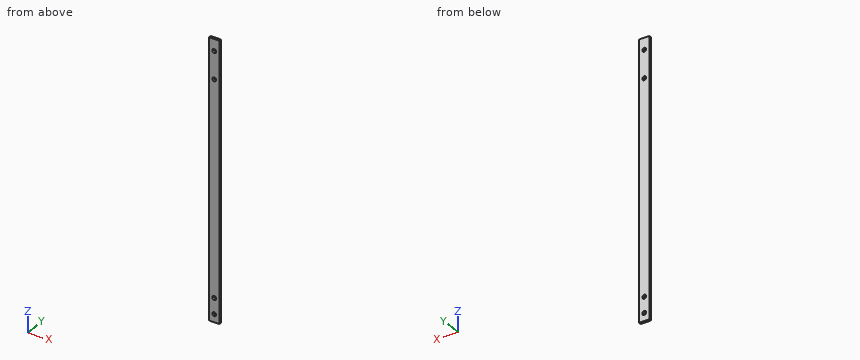
```python
from build123d import *

# Parameters (mm, degrees)
F0_W     = 13
F0_H     = 350
F1_DEPTH = 3
F3_DEPTH = 3
F5_DEPTH = 25
F7_DEPTH = 25
F8_DEPTH = 25


with BuildPart() as f1:
    # F0 (on Front) → F1 (new body)
    with BuildSketch(Plane.XZ):
        Rectangle(F0_W, F0_H)
    extrude(amount=F1_DEPTH)

    # F2 (on face) → F3 (cut)
    with BuildSketch(Plane.XZ.offset(3)):
        with BuildLine():
            ThreePointArc((2.5, 160), (1.767766953, 161.767766953), (0, 162.5))
            ThreePointArc((0, 162.5), (-1.767766953, 158.232233047), (2.5, 160))
        make_face()
    extrude(amount=-F3_DEPTH, mode=Mode.SUBTRACT)

    # F4 (on face) → F5 (cut)
    with BuildSketch(Plane.XZ.offset(3)):
        with BuildLine():
            ThreePointArc((2.5, -145), (-1.767766953, -143.232233047), (0, -147.5))
            ThreePointArc((0, -147.5), (1.767766953, -146.767766953), (2.5, -145))
        make_face()
    extrude(amount=-F5_DEPTH, mode=Mode.SUBTRACT)

    # F6 (on face) → F7 (cut)
    with BuildSketch(Plane.XZ.offset(3)):
        with BuildLine():
            ThreePointArc((2.5, 125), (1.767766953, 126.767766953), (0, 127.5))
            ThreePointArc((0, 127.5), (-1.767766953, 123.232233047), (2.5, 125))
        make_face()
    extrude(amount=-F7_DEPTH, mode=Mode.SUBTRACT)

    # F4 (on face) → F8 (cut)
    with BuildSketch(Plane.XZ.offset(3)):
        with BuildLine():
            ThreePointArc((0, -162.5), (-2.5, -165), (0, -167.5))
            Line((0, -167.5), (0, -165))
            Line((0, -165), (0, -162.5))
        make_face()
        with BuildLine():
            ThreePointArc((2.5, -145), (-1.767766953, -143.232233047), (0, -147.5))
            ThreePointArc((0, -147.5), (1.767766953, -146.767766953), (2.5, -145))
        make_face()
        with BuildLine():
            Line((0, -165), (0, -167.5))
            ThreePointArc((0, -167.5), (1.767766953, -166.767766953), (2.5, -165))
            ThreePointArc((2.5, -165), (1.767766953, -163.232233047), (0, -162.5))
            Line((0, -162.5), (0, -165))
        make_face()
    extrude(amount=-F8_DEPTH, mode=Mode.SUBTRACT)


solid = f1.part
```
Can you work these out from the model? Positions are in its coordinate system, mm. Round coordinates to 2 decimals unless told otherwise and drop trailing zeros. Loops run counter-clockwise (first coordinate to the right, second up) from the corner with the lowest first, then second, coordinate; pieces in that order, holes last. Notation, with made-up numbers: (54.25, 48.25) -> (59.25, 48.25) arc R12 cw to (59.25, 59.25) -> close; hole circle Ø2 at (75.5, 57.5). An arc over 180 degrees is marked (long way). One line per item, written item: value. Start each with the question number.
1. If I drill on probe 1 along Z at (x, y) = (-0.5, -0.5); probe 2 along X at (y, z) = (-1.85, 125); probe 3 along Z at (x, y) = (1.75, -0.55), over which ranges is the centre line in solid material (lowest first)?
2. For pin 1 (4 mm diameter, centred on x = 0, z = 160, fed in from -Y), with a flat end and sliding along its axis, tell me the tip position at first contact or that it passes through.
3. If we section it at A-A, the plane y = -1.2: Write out the boundary of the cut face in (x, z).
Calculated:
1. probe 1: z = -175 to -167.45, -162.55 to -147.45, -142.55 to 122.55, 127.45 to 157.55, 162.45 to 175
1. probe 2: x = -6.5 to -2.5, 2.5 to 6.5
1. probe 3: z = -175 to -166.79, -163.21 to -146.79, -143.21 to 123.21, 126.79 to 158.21, 161.79 to 175
2. pin 1: passes through
3. outline: (-6.5, -175) -> (6.5, -175) -> (6.5, 175) -> (-6.5, 175) -> close; hole circle Ø5 at (0, -165); hole circle Ø5 at (0, -145); hole circle Ø5 at (0, 125); hole circle Ø5 at (0, 160)
